from build123d import *

# Parameters (mm, degrees)
SKETCH1_W           = 23.330000076
SKETCH1_H           = 17.539999972
BOSS_EXTRUDE1_DEPTH = 2
BOSS_EXTRUDE2_DEPTH = 5.08
SKETCH3_W           = 7.62
SKETCH3_H           = 12.7
BOSS_EXTRUDE3_DEPTH = 5.08
SKETCH4_R           = 6.858
CUT_EXTRUDE2_DEPTH  = 29.688494264
BOSS_EXTRUDE4_DEPTH = 12.7
SKETCH6_R           = 1.7
CUT_EXTRUDE3_DEPTH  = 34.67462964


with BuildPart() as part:
    # Sketch1 → Boss-Extrude1 (new body)
    with BuildSketch(Plane(origin=(0, 0, 0), x_dir=(1, 0, 0), z_dir=(0, 1, 0))):
        with Locations((11.665000038, 8.769999986)):
            Rectangle(SKETCH1_W, SKETCH1_H)
    extrude(amount=BOSS_EXTRUDE1_DEPTH)

    # Sketch2 → Boss-Extrude2 (add)
    with BuildSketch(Plane(origin=(0, 2, 0), x_dir=(1, 0, 0), z_dir=(0, 1, 0))):
        Polygon((1.27, 1.778), (1.27, 16.269999972), (22.060000076, 16.269999972), (22.060000076, 1.778), (20.790000076, 1.778), (20.790000076, 14.999999972), (2.54, 14.999999972), (2.54, 1.778), align=None)
    extrude(amount=BOSS_EXTRUDE2_DEPTH)

    # Sketch3 → Boss-Extrude3 (add)
    with BuildSketch(Plane.XZ):
        with Locations((11.665000038, -8.769999986)):
            Rectangle(SKETCH3_W, SKETCH3_H)
    extrude(amount=BOSS_EXTRUDE3_DEPTH)

    # Sketch4 → Cut-Extrude2 (cut, through all)
    with BuildSketch(Plane.XY.offset(-2.419999986)):
        with Locations((11.665000038, -10.782285857)):
            Circle(SKETCH4_R)
    extrude(amount=-CUT_EXTRUDE2_DEPTH, mode=Mode.SUBTRACT)

    # Sketch5 → Boss-Extrude4 (add)
    with BuildSketch(Plane.XY.offset(-2.419999986)):
        with BuildLine():
            ThreePointArc((15.475000038, -5.08), (18.249533344, -10.450286665), (15.475000038, -15.820573329))
            Line((15.475000038, -15.820573329), (15.475000038, -17.026912436))
            Line((15.475000038, -17.026912436), (15.475000038, -23.440573329))
            Line((15.475000038, -23.440573329), (16.491000038, -23.440573329))
            Line((16.491000038, -23.440573329), (16.491000038, -16.322069234))
            ThreePointArc((16.491000038, -16.322069234), (19.240344357, -9.832010848), (15.475000038, -3.873660893))
            Line((15.475000038, -3.873660893), (15.475000038, -5.08))
        make_face()
        with BuildLine():
            ThreePointArc((8.006925979, -15.925190594), (5.081112714, -10.542517711), (7.855000038, -5.08))
            Line((7.855000038, -5.08), (7.855000038, -3.873660893))
            ThreePointArc((7.855000038, -3.873660893), (4.08236068, -9.929050728), (6.990925979, -16.443711247))
            Line((6.990925979, -16.443711247), (6.990925979, -23.545190594))
            Line((6.990925979, -23.545190594), (8.006925979, -23.545190594))
            Line((8.006925979, -23.545190594), (8.006925979, -17.112613639))
            Line((8.006925979, -17.112613639), (8.006925979, -15.925190594))
        make_face()
    extrude(amount=-BOSS_EXTRUDE4_DEPTH)

    # Sketch6 → Cut-Extrude3 (cut, through all)
    with BuildSketch(Plane(origin=(16.491000038, 0, 0), x_dir=(0, 0, -1), z_dir=(1, 0, 0))):
        with Locations(Location((8.769999986, -19.881321281, 0), (0, 0, 270))):
            Circle(SKETCH6_R)
    extrude(amount=-CUT_EXTRUDE3_DEPTH, mode=Mode.SUBTRACT)


solid = part.part
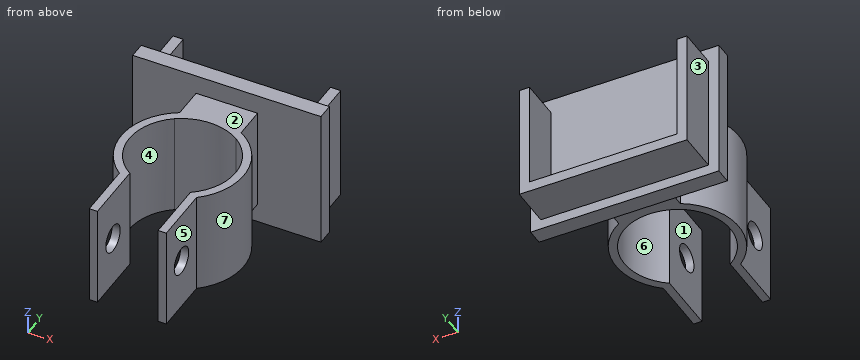
For this review, take the finished solid that the model builds, in its own axes (mm). Face numbers are marked on the shaded views. A direction names the side the tool comes from. Coordinates: 2 decimals unless noted, no trailing zeros. Order: outer loops, then holes, each group sorted by start corner. A loop starts at its lowest first (then second) coordinate and runs counter-clockwise, first axis right, second up. Notation, with made-up numbers: (54, 39.25) - (98, 39.25) arc R21 ccw to (98, 52.25) - close; hole circle Ø4 at (19.5, -37.75). An arc over 180 degrees is marked (long way). Answer as CSV lines item,"result". Start each with the question number.
1) Machinability: for the marked faces 1, 2, 3 and 4, which of the approach directions +Z, -Z, +X, -X, +Y, -Y give a long, thin tool a straight path to every point of the face, cutting with its end or side? Answer none if there is none.
2) Add section B-B (y = -19). State the section outline as (x, z) points (3 decimals).
3) Add section D-D (z = -14.5). State the section outline as (x, y) points (3 decimals), then the cut area to 3 significant figures.
4) Add section A-A (z = -8.77). Count the separate pieces of the cut face and the enclosed holes in it, then the cut area to 3 significant figures.
5) Draft analysis for pull direction Y (two halves, no side actions). For the marked faces 5, 6 and 7, state which applies: +Y half, -Y half, draft (parallel to the pull), parting line (faces both ways), or undercut.
6) To check wall thickness, follow line 1 along X through (y, z) = (-19.5, -7) (3 decimals); line 2 along X through (y, z) = (4, -13); line 3 along Y through (x, z) = (2.25, -15). State the ranges of each line that lie inside material, in increasing order. Write a range as [from, to].
7) Add section C-C (x = 21.5). State the section outline as (y, z) points, then the cut area to 3 significant figures.
8) Insertion check: P1, Ø10, axis at y = -2, z = -7.5, coming from the -X side; P2, Ø0.6, axis at x = 21, y = 5.5, coming from the +Z side; P3, Ø6, axis at y = -20.5, z = -3, coming from the -X side; P4, Ø1.9, axis at y = -1.5, z = -9.5, coming from the +X side (3 decimals). Each pin has a flat end and moves straight along its axis. Give the tip position at first contact, or say it passes through.
Result:
1,face 1,"+Z, -Z, -Y"
1,face 2,"+Z, +X, -X, -Y"
1,face 3,"+Z, -Z, -X, +Y"
1,face 4,"+Z, -Z"
2,outline,"(6.991, -15.12) - (8.007, -15.12) - (8.007, -10.224) - (6.991, -10.224) - close; (6.991, -7.316) - (8.007, -7.316) - (8.007, -2.42) - (6.991, -2.42) - close; (15.475, -15.12) - (16.491, -15.12) - (16.491, -10.224) - (15.475, -10.224) - close; (15.475, -7.316) - (16.491, -7.316) - (16.491, -2.42) - (15.475, -2.42) - close"
3,outline,"(0, 0) - (7.855, 0) - (7.855, -3.874) arc R7.601 ccw to (6.991, -16.444) - (6.991, -23.545) - (8.007, -23.545) - (8.007, -15.925) arc R6.585 cw to (7.855, -5.08) arc R6.858 cw to (15.475, -5.08) arc R6.585 cw to (15.475, -15.821) - (15.475, -23.441) - (16.491, -23.441) - (16.491, -16.322) arc R7.601 ccw to (15.475, -3.874) - (15.475, 0) - (23.33, 0) - (23.33, 2) - (22.06, 2) - (22.06, 7.08) - (20.79, 7.08) - (20.79, 2) - (2.54, 2) - (2.54, 7.08) - (1.27, 7.08) - (1.27, 2) - (0, 2) - close"
3,area,"135 mm^2"
4,separate pieces,"3"
4,enclosed holes,"0"
4,area,"128 mm^2"
5,face 5,"draft"
5,face 6,"undercut"
5,face 7,"undercut"
6,line 1,"[6.991, 8.007], [15.475, 16.491]"
6,line 2,"[1.27, 2.54], [20.79, 22.06]"
6,line 3,"[0, 7.08]"
7,outline,"(0, -17.54) - (2, -17.54) - (2, -16.27) - (7.08, -16.27) - (7.08, -1.78) - (2, -1.78) - (2, 0) - (0, 0) - close"
7,area,"109 mm^2"
8,P1,"x = 0"
8,P2,"z = -1.78"
8,P3,"x = 6.99"
8,P4,"x = 15.475"
